Can you work these out from the drawing? Everything is in mm from the part's minimum corner. A direction names the side the tool comes from. Give positions to 0.01 mm unless a question says otherwise; leave off trailing zeros. Write each loop counter-clockwise with the first axis right and the second up, starting at its lowest first coordinate (ties: lowest second). Pieces come first, ordered by that corner, then holes. Notation, with made-up numbers: (-23, 86.25) - (3, 86.25) arc R24 cw to (3, 96.25) - close; hole circle Ø1 at (27.5, 51). An arc over 180 degrees is marked (long way). Answer in a Markdown table with one row per item.
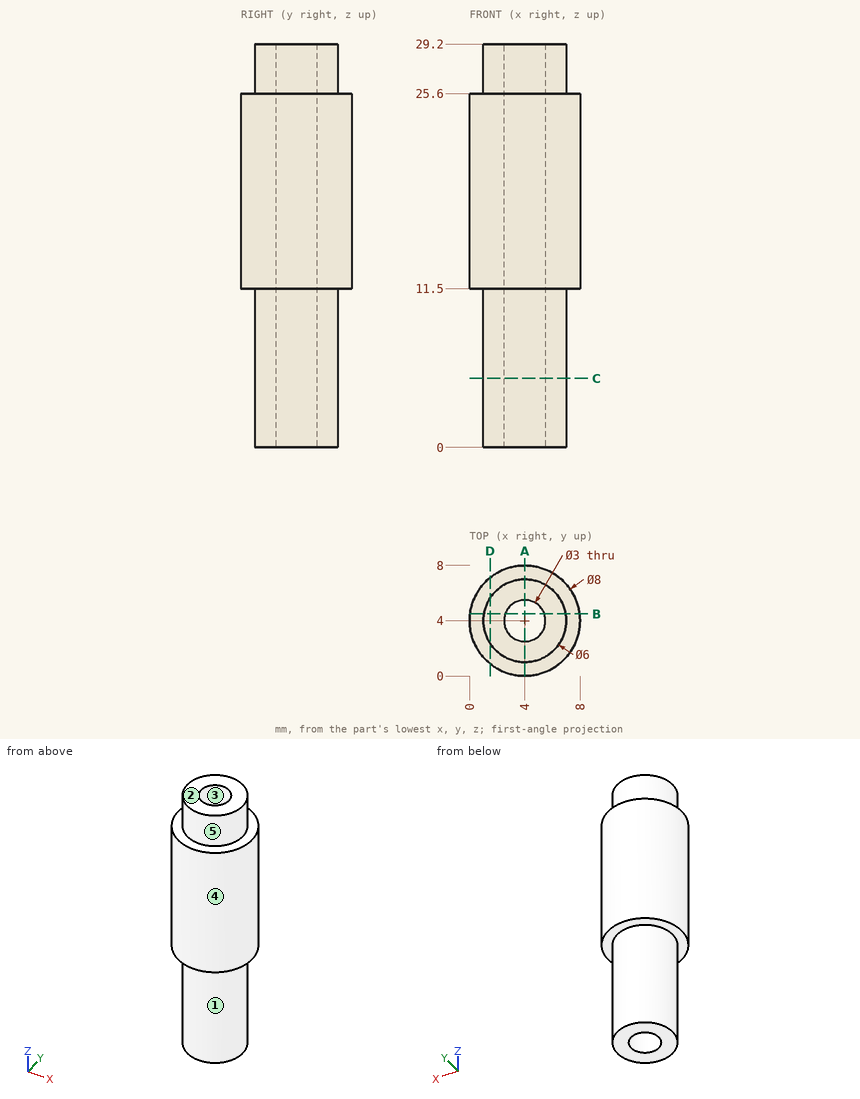
1) Imagine slicing it at D-D (x = 1.5). List the corners of the cut face in (y, z) for me.
Check values:
| item | result |
|---|---|
| outline | (0.88, 11.5) - (2.34, 11.5) - (2.34, 0) - (5.66, 0) - (5.66, 11.5) - (7.12, 11.5) - (7.12, 25.6) - (5.66, 25.6) - (5.66, 29.2) - (2.34, 29.2) - (2.34, 25.6) - (0.88, 25.6) - close |
2) We'd pull the mould along Y, two halves only. Please class the marked faces 1, 2 and 3: +Y half, -Y half, draft (parallel to the pull), parting line (faces both ways), or undercut.
Check values:
| item | result |
|---|---|
| face 1 | parting line |
| face 2 | draft |
| face 3 | undercut |
3) On a 3-axis mill with a long thin cutter (end or side, diameter ignored), from which of +Z, -Z, +X, -X, +Y, -Y can I reach the whole of each face in a straight line? I mean the marked faces 4 and 5. Say none if no direction works.
Check values:
| item | result |
|---|---|
| face 4 | +Z, -Z |
| face 5 | +Z |
4) Imagine slicing it at B-B (y = 4.5). List the corners of the cut face in (x, z) for me.
Check values:
| item | result |
|---|---|
| outline | (0.03, 11.5) - (1.04, 11.5) - (1.04, 0) - (2.59, 0) - (2.59, 29.2) - (1.04, 29.2) - (1.04, 25.6) - (0.03, 25.6) - close; (5.41, 0) - (6.96, 0) - (6.96, 11.5) - (7.97, 11.5) - (7.97, 25.6) - (6.96, 25.6) - (6.96, 29.2) - (5.41, 29.2) - close |
5) Imagine slicing it at A-A (x = 4). List the corners of the cut face in (y, z) for me.
Check values:
| item | result |
|---|---|
| outline | (0, 11.5) - (1, 11.5) - (1, 0) - (2.5, 0) - (2.5, 29.2) - (1, 29.2) - (1, 25.6) - (0, 25.6) - close; (5.5, 0) - (7, 0) - (7, 11.5) - (8, 11.5) - (8, 25.6) - (7, 25.6) - (7, 29.2) - (5.5, 29.2) - close |
6) Imagine slicing it at C-C (z = 5). List the corners of the cut face in (x, y) for me.
Check values:
| item | result |
|---|---|
| outline | circle Ø6 at (4, 4); hole circle Ø3 at (4, 4) |
7) Will this pin go through, and if not, where does the flat tip stop? P1, Ø4, axis at x = 4, y = 4, coming from the +Z side.
Check values:
| item | result |
|---|---|
| P1 | stops at z = 29.2 |
8) If I drill on line 1 (Y direction, x = 4, z = 19.5); line 2 (Y direction, x = 4, z = 9.5), over which ranges is the centre line in solid material (lowest first)?
Check values:
| item | result |
|---|---|
| line 1 | y = 0 to 2.5, 5.5 to 8 |
| line 2 | y = 1 to 2.5, 5.5 to 7 |
